Here's the drawing with two shaded views (mm, measured from the low corner). I have some questions. A direction names the side the tool comes from. Coordinates: 2 decimals unless noted, no trailing zeros. Write each loop counter-clockwise with the first axis right and the second up, starting at its lowest first coordinate (ties: lowest second). Pieces come first, ordered by that corner, then holes.
Item 1: I want a section at C-C on z = 7. Please give me the cut outline in (x, y).
Item 2: Which directions (+Z, -Z, +X, -X, +Y, -Y) give clear straight access to the entire face, cutting with the end or side of a thin tool? Please do the marked faces 4, 5, 6, 7 and 8.
Item 3: For P1, Ø6.5, axis at x = 5.5, z = 5, coming from the -Y side; P2, Ø1.8, axis at x = 36, y = 5, coming from the -Z side; P3, Ø2, axis at x = 6.5, y = 4, coming from the -Z side; P4, Ø4, axis at x = 19, z = 4, coming from the +Y side, each with a flat end and sliding along its axis, tell me the tip position at first contact or that it passes through.
Item 4: I want a section at B-B on y = 5. Please give me the cut outline in (x, z), then the cut area to 3 significant figures.
Item 5: If I drill on probe 1 along X at (y, z) = (0.7, 7); probe 2 along X at (y, z) = (3.75, 9.75); probe 3 along Z at (x, y) = (7, 3.5), over which ranges is the centre line in solid material (lowest first)?
Item 6: I want a section at D-D on y = 1. Please give me the cut outline in (x, z), then the cut area to 3 significant figures.
Item 7: Thinking about a two-plate mould opening in Z: for the marked faces 1, 2 and 3, which applies, +Z half, -Z half, draft (parallel to the pull), parting line (faces both ways), or undercut?
Item 8: I want a section at A-A on x = 14.5. Please give me the cut outline in (y, z).
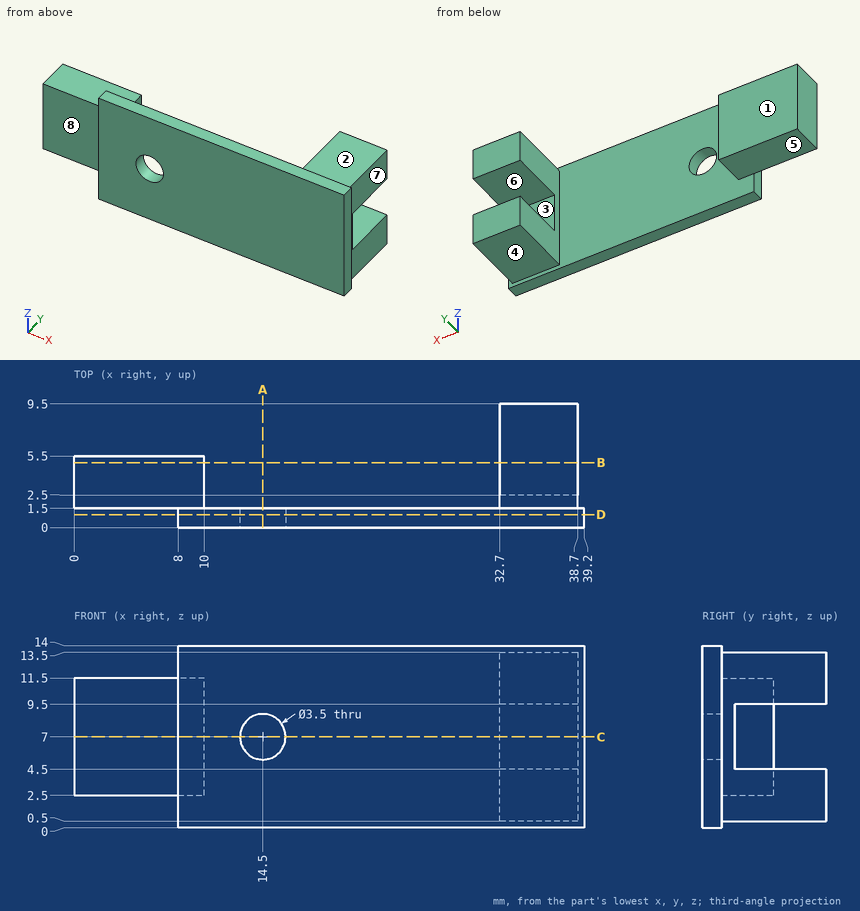
Response values:
1. outline: (0, 1.5) - (8, 1.5) - (8, 0) - (12.75, 0) - (12.75, 1.5) - (10, 1.5) - (10, 5.5) - (0, 5.5) - close; (16.25, 0) - (39.2, 0) - (39.2, 1.5) - (38.7, 1.5) - (38.7, 2.5) - (32.7, 2.5) - (32.7, 1.5) - (16.25, 1.5) - close
2. face 4: -Z, +X, -X, +Y
2. face 5: -Z, -X, +Y
2. face 6: +X, +Y
2. face 7: +Z, -Z, +X, +Y
2. face 8: +Z, -Z, -X, -Y
3. P1: stops at y = 0
3. P2: stops at z = 0.5
3. P3: stops at z = 2.5
3. P4: stops at y = 1.5
4. outline: (0, 2.5) - (10, 2.5) - (10, 11.5) - (0, 11.5) - close; (32.7, 0.5) - (38.7, 0.5) - (38.7, 4.5) - (32.7, 4.5) - close; (32.7, 9.5) - (38.7, 9.5) - (38.7, 13.5) - (32.7, 13.5) - close
4. area: 138 mm2
5. probe 1: x = 8 to 12.75, 16.25 to 39.2
5. probe 2: x = 0 to 10, 32.7 to 38.7
5. probe 3: z = 2.5 to 11.5
6. outline: (8, 0) - (39.2, 0) - (39.2, 14) - (8, 14) - close; hole circle Ø3.5 at (14.5, 7)
6. area: 427 mm2
7. face 1: draft
7. face 2: +Z half
7. face 3: undercut
8. outline: (0, 0) - (1.5, 0) - (1.5, 5.25) - (0, 5.25) - close; (0, 8.75) - (1.5, 8.75) - (1.5, 14) - (0, 14) - close
